Verification items for this drawing (mm, ordinates from the low corner). A direction names the side the tool comes from. Coordinates: 2 decimals unless noted, no trailing zeros. Order: outer loops, then holes, each group sorted by start corner. A loop starts at its lowest first (then second) coordinate and runs counter-clockwise, first axis right, second up. Notation, with made-up numbers: (60, 80.5) -> (111, 80.5) arc R8 ccw to (111, 95.5) -> close; hole circle Ø9 at (-36, 60.25). An arc over 180 degrees is marked (long way). Write each question's results on one line, items separated by ' | '. Start each with the question number.
(1) Go/stop test with flat-tipped pins: pin 1 (5 mm diameter, centred on x = 2.5, z = 6, fed in from +Y); pin 2 (0.5 mm diameter, centred on y = 0.5, z = 1.5, fed in from -X). Record where each tip stops, or that it passes through.
(2) Draft check along X on the marked faces 3, 4, 5 and 6. Enter one of: +X half, -X half, draft (parallel to the pull), parting line (faces both ways), or undercut.
(3) Cross-section at C-C on y = 0.3. Enter the section's corners in (x, z) (1 decimal).
(4) Thickness scan on probe 1 along Z at (x, y) = (2.25, 0.3) (1 decimal); probe 2 along X at (y, z) = (0.9, 4.5); probe 3 along X at (y, z) = (0.8, 5.5) (1 decimal). Record the ranges inside material, lowest first. Write a range as [from, to].
(5) Cross-section at A-A on z = 2. Enter the section's corners in (x, y) (1 decimal).
(6) Cross-section at B-B on x = 3.25. Enter the section's corners in (y, z).
(7) Set-up check for the marked faces 1 and 2: record each of +Z, -Z, +X, -X, +Y, -Y from which the full face is reachable in a straight line by a thin tool's end or side.
(8) Cross-section at D-D on z = 8. Enter the section's corners in (x, y) (1 decimal).
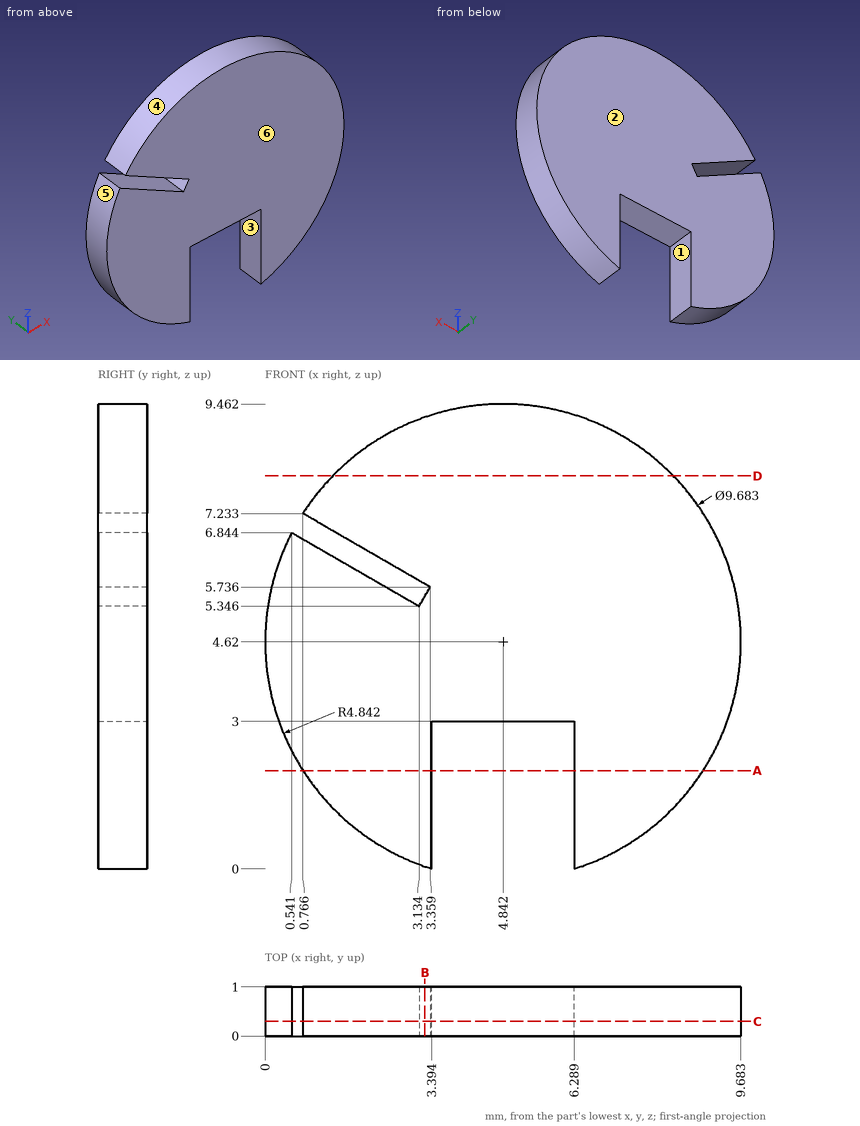
Results are:
1) pin 1: stops at y = 1 | pin 2: stops at x = 0.94
2) face 3: undercut | face 4: parting line | face 5: -X half | face 6: draft
3) outline: (0.5, 6.8) arc R4.8 ccw to (3.4, 0) -> (3.4, 3) -> (6.3, 3) -> (6.3, 0) arc R4.8 ccw (long way) to (0.8, 7.2) -> (3.4, 5.7) -> (3.1, 5.3) -> close
4) probe 1: z = [0.5, 5.9], [6.4, 8.7] | probe 2: x = [0, 9.68] | probe 3: x = [0.1, 2.9], [3.2, 9.6]
5) outline: (0.8, 0) -> (3.4, 0) -> (3.4, 1) -> (0.8, 1) -> close; (6.3, 0) -> (8.9, 0) -> (8.9, 1) -> (6.3, 1) -> close
6) outline: (0, 0.05) -> (1, 0.05) -> (1, 5.55) -> (0, 5.55) -> close; (0, 5.8) -> (1, 5.8) -> (1, 9.19) -> (0, 9.19) -> close
7) face 1: -Z, +Y, -Y | face 2: +Z, -Z, +X, -X, +Y
8) outline: (1.4, 0) -> (8.3, 0) -> (8.3, 1) -> (1.4, 1) -> close
